Autodesk Inventor part; units mm, degrees
ref_plane "Work Plane1" through (0, 0, -144) normal (0, 0, 1) x (1, 0, 0)
ref_plane "XZ Plane" through (0, 0, 0) normal (0, 1, 0) x (-1, 0, 0)
ref_plane "UCS4: YZ Plane" through (0, 0, 0) normal (1, 0, 0) x (0, 1, 0)
sketch "Sketch1" plane through (0, 0, 0) normal (0, 0, 1) x (1, 0, 0)
  line L0 (-20, -20) -> (20, -20)
  line L1 (20, -20) -> (20, 28)
  line L2 (20, 28) -> (-20, 28)
  line L3 (-20, 28) -> (-20, -20)
  line L4 (-20, -20) -> (20, 28) construction
  line L5 (20, -20) -> (-20, 28) construction
  line L6 (0, -29.6) -> (0, 37.6)
  point P0 (0, 0)
  point P1 (0, 4)
  dimension "d0" = 20
  dimension "d1" = 28
  dimension "d2" = 40
extrude "Extrusion1" add sketch "Sketch1" along normal blind 4 and the other way blind 116
sketch "Sketch3" plane through (0, 0, -116) normal (0, 0, -1) x (-1, 0, 0)
  line L0 (-20, -20) -> (20, -20)
  line L1 (20, -20) -> (20, 20)
  line L2 (20, 20) -> (-20, 20)
  line L3 (-20, 20) -> (-20, -20)
  line L4 (-20, -20) -> (20, 20) construction
  line L5 (20, -20) -> (-20, 20) construction
  line L6 (0, -29.6) -> (0, 37.6)
  line L7 (-20, -20) -> (20, -20)
  line L8 (20, -20) -> (20, 28)
  line L9 (20, 28) -> (-20, 28)
  point P0 (0, 0)
  point P1 (0, 0)
  point P2 (0, 0)
  dimension "d16" = 8
extrude "Extrusion3" add sketch "Sketch3" along normal blind 96 contours L3 L2 L6 L0 | L6 L2 L1 L0
ref_plane "Work Plane1" through (0, 0, -144) normal (0, 0, 1) x (1, 0, 0)
sketch "Sketch4" plane through (0, 0, -144) normal (0, 0, 1) x (1, 0, 0)
  circle A0 centre (0, 0) radius 30
  dimension "d20" = 60
extrude "Extrusion4" add sketch "Sketch4" along normal mid plane 14
sketch "Sketch5" plane through (0, 0, -212) normal (0, 0, -1) x (-1, 0, 0)
  circle A0 centre (0, 0) radius 30
  dimension "d23" = 60
extrude "Extrusion5" add sketch "Sketch5" along normal blind 8
ref_plane "UCS4: YZ Plane" through (0, 0, 0) normal (1, 0, 0) x (0, 1, 0)
ref_plane "UCS4: XZ Plane" through (0, 0, 0) normal (0, 1, 0) x (0, 0, 1)
ref_plane "UCS4: XY Plane" through (0, 0, 0) normal (0, 0, 1) x (1, 0, 0)
properties part number "link_4"
Model file for the job. Use its own axes, mm. A direction names the side the tool comes from. Round coordinates to 2 decimals unless told otherwise and drop trailing zeros. Order: outer loops, then holes, each group sorted by start corner. A loop starts at its lowest first (then second) coordinate and runs counter-clockwise, first axis right, second up. Notation, with made-up numbers: M 22.5,45.25 L 35.5,45.25 A16 cw 35.5,52.25 Z; hole C 43.25,77 d6. An arc over 180 degrees is marked long. Use CSV: the item, a comma, the result in double quotes.
Item 1: Pin check, flat tips, straight feed: pin 1 (20 mm diameter, centred on x = -0.5, z = -168, fed in from -Y); pin 2 (14.5 mm diameter, centred on y = -4.5, z = -60, fed in from -X); pin 3 (10 mm diameter, centred on x = 17, z = -58, fed in from +Y). Stop position of each tip, or through.
Worked answers:
pin 1,"y = -20"
pin 2,"x = -20"
pin 3,"y = 28"
Item 2: Probe probe 1 along Z at (x, y) = (13.5, 25); probe 2 along Z at (x, y) = (26.5, 6); probe 3 along Y at (x, z) = (6, -47). List the from-to ranges inside material, lowest first.
Worked answers:
probe 1,"-220 to -212, -151 to -137, -116 to 4"
probe 2,"-220 to -212, -151 to -137"
probe 3,"-20 to 28"
Item 3: Saw through at A-A (y = 24). List the corners of the cut face in (x, z), plus the area to 3 significant figures.
Worked answers:
outline,"M -20,-116 L 20,-116 L 20,4 L -20,4 Z; M -18,-220 L 18,-220 L 18,-212 L -18,-212 Z; M -18,-151 L 18,-151 L 18,-137 L -18,-137 Z"
area,"5,590 mm²"
Item 4: Which spindle directions (+Z, -Z, +X, -X, +Y, -Y) get a long thin tool onto all of the face, cutting with end or side? Do faces 5 (the face through (0, -20, -182)), 6 (the face through (20, 4, -67)), 7 (the face through (0, 20, -126)), 8 (the face through (-20, 0, -182)). Say none if no direction does.
Worked answers:
face 5,"+X, -X, -Y"
face 6,"+Z, +X, +Y, -Y"
face 7,"+X, -X, +Y"
face 8,"-X, +Y, -Y"
Item 5: Pull direction Z, two halves, no side cores. Call faces 1 (the face through (0, 24, -116)), 2 (the face through (-22, 2, -137)), 3 (the face through (-20, 4, -67)), 4 (the face through (0, 0, -220)): released by +Z, released by -Z, zero draft, split by the parting line, or undercut.
Worked answers:
face 1,"undercut"
face 2,"undercut"
face 3,"zero draft"
face 4,"released by -Z"
Item 6: Saw through at D-D (y = 0). List the corners of the cut face in (x, z), plus the area to 3 significant figures.
Worked answers:
outline,"M -30,-220 L 30,-220 L 30,-212 L 20,-212 L 20,-151 L 30,-151 L 30,-137 L 20,-137 L 20,4 L -20,4 L -20,-137 L -30,-137 L -30,-151 L -20,-151 L -20,-212 L -30,-212 Z"
area,"9,400 mm²"
Item 7: Saw through at B-B (x = -23). List the corners of the cut face in (y, z), plus the area to 4 significant figures.
Worked answers:
outline,"M -19.26,-220 L 19.26,-220 L 19.26,-212 L -19.26,-212 Z; M -19.26,-151 L 19.26,-151 L 19.26,-137 L -19.26,-137 Z"
area,"847.5 mm²"
Item 8: Saw through at C-C (x = 0). List the corners of the cut face in (y, z).
Worked answers:
outline,"M -30,-220 L 30,-220 L 30,-212 L 20,-212 L 20,-151 L 30,-151 L 30,-137 L 20,-137 L 20,-116 L 28,-116 L 28,4 L -20,4 L -20,-137 L -30,-137 L -30,-151 L -20,-151 L -20,-212 L -30,-212 Z"
